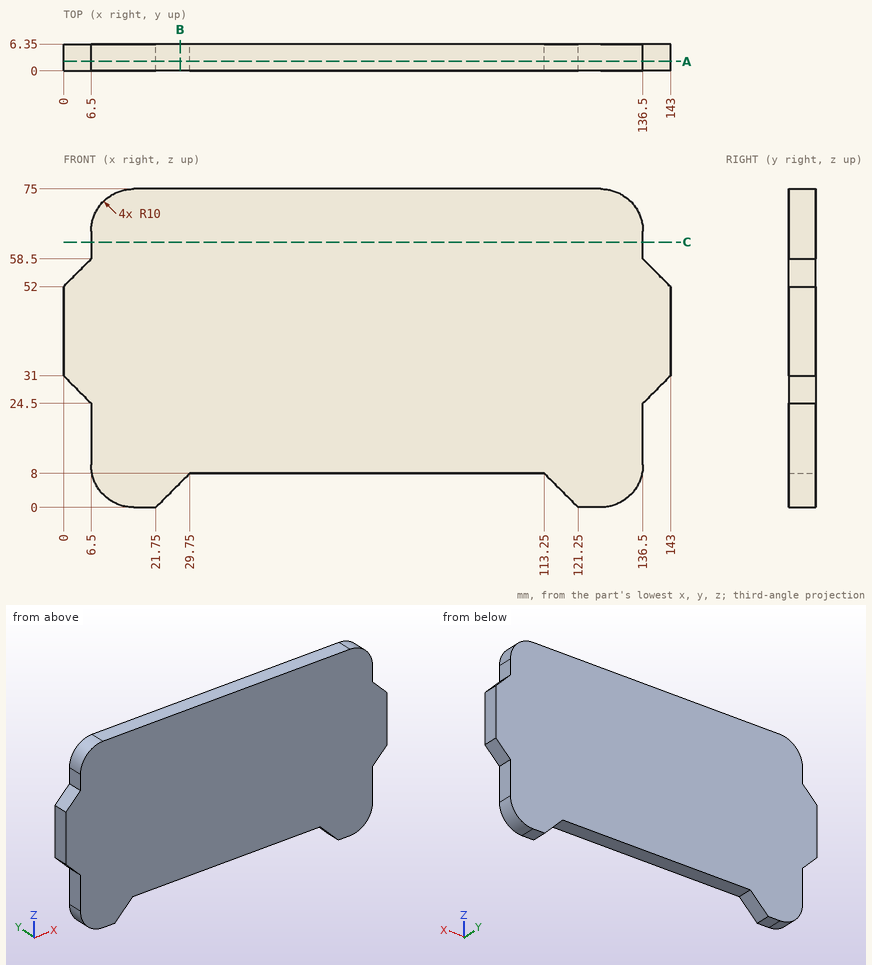
The figure shows three views and two pictorial views of one solid part (mm, origin at its lowest corner). Answer the questions. Give positions to 0.01 mm unless a question says otherwise; leave off trailing zeros. Write each loop counter-clockwise with the first axis right and the second up, starting at its lowest first coordinate (ties: lowest second). Pieces come first, ordered by that corner, then holes. Notation, with made-up numbers: (86, -36.75) - (103, -36.75) arc R14 cw to (103, -27.75) - close; hole circle Ø9 at (46.25, 47.5). An arc over 180 degrees is marked (long way). Use one line per item in the form item = value.
1. Each of these flat-tipped pins is pushed along its axis until it touches: pin 1 Ø3 at (y, z) = (4, 19) entering from +X; pin 2 Ø3 at (x, y) = (61, 2) entering from -Z; pin 3 Ø1.5 at (x, y) = (22, 3.5) entering from -Z; pin 4 Ø1 at (y, z) = (1, 58) entering from +X. Where does it stop, or does it pass through?
Filled in:
pin_1 = 136.5
pin_2 = 8
pin_3 = 0
pin_4 = 137.5
2. Consider L1, parallel to Z at x = 112.5, y = 3.25; L2, parallel to X at y = 0.75, z = 58.5; L3, parallel to X at y = 3.75, z = 4. Determine where each line is inside the solid, lowest interval first.
Filled in:
L1 = 8 to 75
L2 = 6.5 to 136.5
L3 = 8.5 to 25.75, 117.25 to 134.5
3. A cutting plane is placed at B-B (x = 27.5). Write down the section's boundary in (y, z).
Filled in:
outline = (0, 5.75) - (6.35, 5.75) - (6.35, 75) - (0, 75) - close
4. A cutting plane is placed at C-C (z = 62.5). Write down the section's boundary in (x, y), and give its area (4 significant figures).
Filled in:
outline = (6.5, 0) - (136.5, 0) - (136.5, 6.35) - (6.5, 6.35) - close
area = 825.5 mm^2
5. A cutting plane is placed at A-A (y = 2.25). Write down the section's boundary in (x, z), and give its area (3 significant figures).
Filled in:
outline = (0, 31) - (6.5, 24.5) - (6.5, 10) arc R10 ccw to (16.5, 0) - (21.75, 0) - (29.75, 8) - (113.25, 8) - (121.25, 0) - (126.5, 0) arc R10 ccw to (136.5, 10) - (136.5, 24.5) - (143, 31) - (143, 52) - (136.5, 58.5) - (136.5, 65) arc R10 ccw to (126.5, 75) - (16.5, 75) arc R10 ccw to (6.5, 65) - (6.5, 58.5) - (0, 52) - close
area = 9,290 mm^2
